```python
from build123d import *

# Parameters (mm, degrees)
F2_R     = 1.55
F3_DEPTH = 5.001
F4_R     = 15
F5_R     = 2


with BuildPart() as f1:
    # F0 (on Front) → F1 (revolve)
    with BuildSketch(Plane.XZ):
        Polygon((0, 0), (47.5, 0), (47.5, 2), (43.5, 2), (43.5, 5), (40.8, 5), (40.8, 2), (36.8, 2), (36.8, 5), (34.1, 5), (34.1, 2), (30.1, 2), (30.1, 5), (27.4, 5), (27.4, 2), (23.4, 2), (23.4, 5), (0, 5), align=None)
    revolve(axis=Axis((0, 0, 0.333373), (0, 0, -1)))

    # F2 (on face) → F3 (cut, through all)
    with BuildSketch(Plane.XY.offset(5)):
        with BuildLine():
            ThreePointArc((3.427323, -0.824065), (3.05274, 1.7625), (1, 3.380181))
            Line((1, 3.380181), (1, 5.91608))
            ThreePointArc((1, 5.91608), (0, 6), (-1, 5.91608))
            Line((-1, 5.91608), (-1, 3.380181))
            ThreePointArc((-1, 3.380181), (-3.05274, 1.7625), (-3.427323, -0.824065))
            Line((-3.427323, -0.824065), (-5.623475, -2.092014))
            ThreePointArc((-5.623475, -2.092014), (-5.196152, -3), (-4.623475, -3.824065))
            Line((-4.623475, -3.824065), (-2.427323, -2.556116))
            ThreePointArc((-2.427323, -2.556116), (0, -3.525), (2.427323, -2.556116))
            Line((2.427323, -2.556116), (4.623475, -3.824065))
            ThreePointArc((4.623475, -3.824065), (5.196152, -3), (5.623475, -2.092014))
            Line((5.623475, -2.092014), (3.427323, -0.824065))
        make_face()
        with BuildLine():
            ThreePointArc((-6.974937, 0.59182), (-6.062178, 3.5), (-4, 5.744563))
            Line((-4, 5.744563), (-4, 19.595918))
            ThreePointArc((-4, 19.595918), (-17.320508, 10), (-18.970563, -6.333857))
            Line((-18.970563, -6.333857), (-6.974937, 0.59182))
        make_face()
        with BuildLine():
            Line((4, 19.595918), (4, 5.744563))
            ThreePointArc((4, 5.744563), (6.062178, 3.5), (6.974937, 0.59182))
            Line((6.974937, 0.59182), (18.970563, -6.333857))
            ThreePointArc((18.970563, -6.333857), (17.320508, 10), (4, 19.595918))
        make_face()
        with Locations((0, 16)):
            Circle(F2_R)
        with BuildLine():
            ThreePointArc((2.974937, -6.336383), (0, -7), (-2.974937, -6.336383))
            Line((-2.974937, -6.336383), (-14.970563, -13.262061))
            ThreePointArc((-14.970563, -13.262061), (0, -20), (14.970563, -13.262061))
            Line((14.970563, -13.262061), (2.974937, -6.336383))
        make_face()
        with Locations((-13.856406, -8)):
            Circle(F2_R)
        with Locations((13.856406, -8)):
            Circle(F2_R)
    extrude(amount=-F3_DEPTH, mode=Mode.SUBTRACT)

    # F4
    f4_edges = [f1.edges().sort_by_distance(p)[0] for p in [
        (4, 5.744563, 2.5),
        (6.974937, 0.59182, 2.5),
        (-2.974937, -6.336383, 2.5),
        (2.974937, -6.336383, 2.5),
        (-4, 5.744563, 2.5),
        (-6.974937, 0.59182, 2.5),
    ]]
    fillet(f4_edges, radius=F4_R)

    # F5
    f5_edges = [f1.edges().sort_by_distance(p)[0] for p in [
        (-4, 19.595918, 2.5),
        (4, 19.595918, 2.5),
        (-18.970563, -6.333857, 2.5),
        (-14.970563, -13.262061, 2.5),
        (14.970563, -13.262061, 2.5),
        (18.970563, -6.333857, 2.5),
    ]]
    fillet(f5_edges, radius=F5_R)


solid = f1.part
```
Could you check a few things on this model? Use its own coordinates, in mm. A direction names the side the tool comes from. Coordinates: 2 decimals unless noted, no trailing zeros. Write each loop counter-clockwise with the first axis right and the second up, starting at its lowest first coordinate (ties: lowest second). Pieces come first, ordered by that corner, then holes. Notation, with made-up numbers: (55, 1) - (107, 1) arc R17 ccw to (107, 34) - close; hole circle Ø11 at (20, 82.5). An arc over 180 degrees is marked (long way). Use a Markdown table: item, result.
Q1. Imagine slicing it at C-C (x = -32). List the corners of the cut face in (y, z) for me, and give its area (3 significant figures).
Geometry check:
| item | result |
|---|---|
| outline | (-35.1, 0) - (35.1, 0) - (35.1, 2) - (29.47, 2) - (29.47, 5) - (25.31, 5) - (25.31, 2) - (18.17, 2) - (18.17, 5) - (11.78, 5) - (11.78, 2) - (-11.78, 2) - (-11.78, 5) - (-18.17, 5) - (-18.17, 2) - (-25.31, 2) - (-25.31, 5) - (-29.47, 5) - (-29.47, 2) - (-35.1, 2) - close |
| area | 204 mm2 |
Q2. Imagine slicing it at A-A (z = 3.7). Count the separate pieces of the cut face and the enclosed holes in it, and give its area (3 significant figures).
Geometry check:
| item | result |
|---|---|
| separate pieces | 4 |
| enclosed holes | 10 |
| area | 2,690 mm2 |
Q3. Imagine slicing it at B-B (y = 25.5). List the corners of the cut face in (x, z) for me.
Geometry check:
| item | result |
|---|---|
| outline | (-40.07, 0) - (40.07, 0) - (40.07, 2) - (35.24, 2) - (35.24, 5) - (31.85, 5) - (31.85, 2) - (26.53, 2) - (26.53, 5) - (22.64, 5) - (22.64, 2) - (15.99, 2) - (15.99, 5) - (10.03, 5) - (10.03, 2) - (-10.03, 2) - (-10.03, 5) - (-15.99, 5) - (-15.99, 2) - (-22.64, 2) - (-22.64, 5) - (-26.53, 5) - (-26.53, 2) - (-31.85, 2) - (-31.85, 5) - (-35.24, 5) - (-35.24, 2) - (-40.07, 2) - close |
Q4. Which directions (+Z, -Z, +X, -X, +Y, -Y) give clear straight access to the entire face, cutting with the end or side of a thin tool? Please do faces 1 (the cylindrical face through (4.506, 7.227, 2.465)), 2 (the cylindrical face through (-20.195, -18.518, 3.479)), 3 (the flat face through (5, 0, 5)).
Geometry check:
| item | result |
|---|---|
| face 1 | +Z, -Z |
| face 2 | +Z |
| face 3 | +Z, +X, -X, +Y, -Y |
Q5. I'm going to push flat-ended pins straight in: pin 1 Ø1 at (y, z) = (14.5, 3) entering from -X; pin 2 Ø2 at (x, y) = (-25.5, 25.5) entering from -Z; pin 3 Ø3 at (y, z) = (4.5, 1.5) entering from -X; pin 4 Ø1.5 at (y, z) = (9.5, 4) entering from -X. Where does each tip first touch, or does it pass through?
Geometry check:
| item | result |
|---|---|
| pin 1 | stops at x = -41.19 |
| pin 2 | stops at z = 0 |
| pin 3 | stops at x = -47.41 |
| pin 4 | stops at x = -42.61 |
Q6. Thinking about a two-plate mould opening in X: for faces 4 (the cylindrical face through (18.558, -5.094, 2.465)), 5 (the flat face through (1, 10, 0)), which applies, +X half, -X half, draft (parallel to the pull), parting line (faces both ways), or undercut?
Geometry check:
| item | result |
|---|---|
| face 4 | undercut |
| face 5 | draft |
Q7. Imagine slicing it at D-D (y = -25). List the corners of the cut face in (x, z) for me, and give its area (3 significant figures).
Geometry check:
| item | result |
|---|---|
| outline | (-40.39, 0) - (40.39, 0) - (40.39, 2) - (35.6, 2) - (35.6, 5) - (32.24, 5) - (32.24, 2) - (27, 2) - (27, 5) - (23.19, 5) - (23.19, 2) - (16.76, 2) - (16.76, 5) - (11.21, 5) - (11.21, 2) - (-11.21, 2) - (-11.21, 5) - (-16.76, 5) - (-16.76, 2) - (-23.19, 2) - (-23.19, 5) - (-27, 5) - (-27, 2) - (-32.24, 2) - (-32.24, 5) - (-35.6, 5) - (-35.6, 2) - (-40.39, 2) - close |
| area | 238 mm2 |
Q8. Please list where these lines run through material, in increasing order: L1, parallel to Y at x = 24.5, z = 2.4 (3 decimals); L2, parallel to Z at x = 19.5, y = 40; L3, parallel to Y at x = -12, z = 0.5.
Geometry check:
| item | result |
|---|---|
| L1 | y = -35.944 to -32.625, -27.459 to -23.718, -17.486 to -12.268, 12.268 to 17.486, 23.718 to 27.459, 32.625 to 35.944 |
| L2 | z = 0 to 2 |
| L3 | y = -45.96 to -16, -11.55 to -2.31, 16 to 45.96 |
